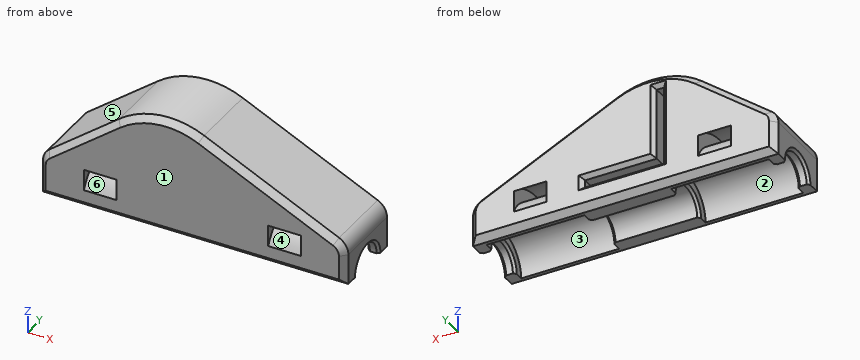
from build123d import *

# Parameters (mm, degrees)
PAD_DEPTH       = 10
SKETCH001_R     = 5
POCKET_DEPTH    = 75.001
POCKET001_DEPTH = 15
SKETCH003_W     = 24
SKETCH003_H     = 7.6
SKETCH003_W_2   = 8
SKETCH003_H_2   = 3
CHAMFER_SIZE    = 0.6
FILLET_R        = 20
FILLET001_R     = 4
CHAMFER001_SIZE = 1.5
CHAMFER002_SIZE = 1


with BuildPart() as part:
    # Sketch → Pad (new body, symmetric)
    with BuildSketch(Plane.XZ):
        Polygon((-37.5, 0), (37.5, 0), (37.5, 10), (-9, 32), (-37.5, 10), align=None)
    extrude(amount=PAD_DEPTH, both=True)

    # Sketch001 (on Face2 of Pad) → Pocket (cut, through all)
    with BuildSketch(Plane(origin=(37.5, 0, 0), x_dir=(0, 0, 1), z_dir=(1, 0, 0))):
        Circle(SKETCH001_R)
    extrude(amount=-POCKET_DEPTH, mode=Mode.SUBTRACT)

    # Sketch002 (on Face2 of Pocket) → Pocket001 (cut)
    with BuildSketch(Plane(origin=(0, 10, 0), x_dir=(1, 0, 0), z_dir=(0, 1, 0))):
        Polygon((-9.7, -25.4), (-9.7, -6), (9.7, -6), (9.7, -7.8), (-7.9, -7.8), (-7.9, -25.4), align=None)
    extrude(amount=-POCKET001_DEPTH, mode=Mode.SUBTRACT)

    # Sketch003 → Groove (revolve, cut)
    with BuildSketch(Plane.XZ):
        with Locations((-22.636851, 3.8)):
            Rectangle(SKETCH003_W, SKETCH003_H)
        with Locations((22.636851, 3.8)):
            Rectangle(SKETCH003_W, SKETCH003_H)
        with Locations((-22.636851, 12.5)):
            Rectangle(SKETCH003_W_2, SKETCH003_H_2)
        with Locations((22.636851, 12.5)):
            Rectangle(SKETCH003_W_2, SKETCH003_H_2)
    revolve(axis=Axis((0, 0, 0), (1, 0, 0)), mode=Mode.SUBTRACT)

    # Chamfer
    chamfer_edges = [part.edges().sort_by_distance(p)[0] for p in [
        (37.5, 3.535534, 3.535534),
        (34.636851, 0, 5),
        (10.636851, 0, 5),
        (-10.636851, 0, 5),
        (-34.636851, 0, 5),
        (-37.5, 3.535534, 3.535534),
    ]]
    chamfer(chamfer_edges, length=CHAMFER_SIZE)

    # Fillet
    fillet_edges = [part.edges().sort_by_distance(p)[0] for p in [
        (-9, 0, 32),
    ]]
    fillet(fillet_edges, radius=FILLET_R)

    # Fillet001
    fillet001_edges = [part.edges().sort_by_distance(p)[0] for p in [
        (37.5, 0, 10),
        (-37.5, 0, 10),
    ]]
    fillet(fillet001_edges, radius=FILLET001_R)

    # Chamfer001
    chamfer001_edges = [part.edges().sort_by_distance(p)[0] for p in [
        (18.643068, 10, 18.921559),
        (0, 10, 0),
        (18.643068, -10, 18.921559),
        (0, -10, 0),
    ]]
    chamfer(chamfer001_edges, length=CHAMFER001_SIZE)

    # Chamfer002
    chamfer002_edges = [part.edges().sort_by_distance(p)[0] for p in [
        (-9.7, 10, 15.7),
        (-7.9, 10, 16.6),
        (-8.8, 10, 25.4),
        (0, 10, 6),
        (0.9, 10, 7.8),
        (9.7, 10, 6.9),
    ]]
    chamfer(chamfer002_edges, length=CHAMFER002_SIZE)


solid = part.part
Check sheet for the modelled part. Datum: model origin and axes. Units: mm. Face numbers are marked on the shaded views. A direction names the side the tool comes from. Round coordinates to 2 decimals unless told otherwise and drop trailing zeros. Order: outer loops, then holes, each group sorted by start corner. A loop starts at its lowest first (then second) coordinate and runs counter-clockwise, first axis right, second up.
Q1. Cross-section at A-A, the plane x = 6. Enter the section's corners in (y, z), plus the area to 3 significant figures.
Filled sheet:
outline: (-10, 1.5) - (-8.5, 0) - (-5, 0) arc R5 cw to (5, 0) - (8.5, 0) - (10, 1.5) - (10, 5) - (9, 6) - (-5, 6) - (-5, 7.8) - (9, 7.8) - (10, 8.8) - (10, 23.24) - (8.5, 24.9) - (-8.5, 24.9) - (-10, 23.24) - close
area: 426 mm2
Q2. Cross-section at B-B, the plane y = 0. Give the number of separate pieces and of enclosed holes in the cut face, plus the area to 3 significant figures.
Filled sheet:
separate pieces: 1
enclosed holes: 3
area: 933 mm2
Q3. Depth check by flat-ended pin: P1, Ø4, axis at y = 0, z = 4, coming from the +X side; P2, Ø2, axis at y = 2, z = 14.5, coming from the -X side; P3, Ø12, axis at x = -27.5, y = 5.5, coming from the +Z side; P4, Ø7, axis at y = 4.5, z = 16.5, coming from the -X side. Enter the tip coordinate at first touch or a pass-through.
Filled sheet:
P1: stops at x = 37.5
P2: stops at x = -32.97
P3: stops at z = 22.35
P4: stops at x = -33.61
Q4. Scan lines: L1, parallel to X at y = 6, z = 7; L2, parallel to X at y = 3, z = 13; L3, parallel to Z at x = -9, y = 6.75. Record each from-to range of solid material in increasing order.
Filled sheet:
L1: x = -37.5 to -9.7, 9.7 to 37.5
L2: x = -33.61 to -26.64, -18.64 to -9.7, -7.9 to 18.64, 26.64 to 31.16
L3: z = 0 to 6, 25.4 to 28.52
Q5. Draft check along Z on the marked faces 3, 4, 5 and 6. Enter one of: pulls with the +Z half, pulls with the -Z half, needs draft (parallel to the pull), parting line crosses it, or undercut.
Filled sheet:
face 3: pulls with the -Z half
face 4: undercut
face 5: pulls with the +Z half
face 6: undercut
Q6. Set-up check for the marked faces 1 and 2: record each of +Z, -Z, +X, -X, +Y, -Y from which the full face is reachable in a straight line by a thin tool's end or side.
Filled sheet:
face 1: +Z, -Z, +X, -X, -Y
face 2: -Z
